Here's the drawing with two shaded views (mm, measured from the low corner). I have some questions. A direction names the side the tool comes from. Coordinates: 2 decimals unless noted, no trailing zeros. Loops run counter-clockwise (first coordinate to the right, second up) from the corner with the lowest first, then second, coordinate; pieces in that order, holes last. Notation, with made-up numbers: (80, 50.5) - (123, 50.5) arc R21 ccw to (123, 88.5) - close; hole circle Ø2 at (-35.75, 80). An arc over 180 degrees is marked (long way). Use a Markdown table: item, result.
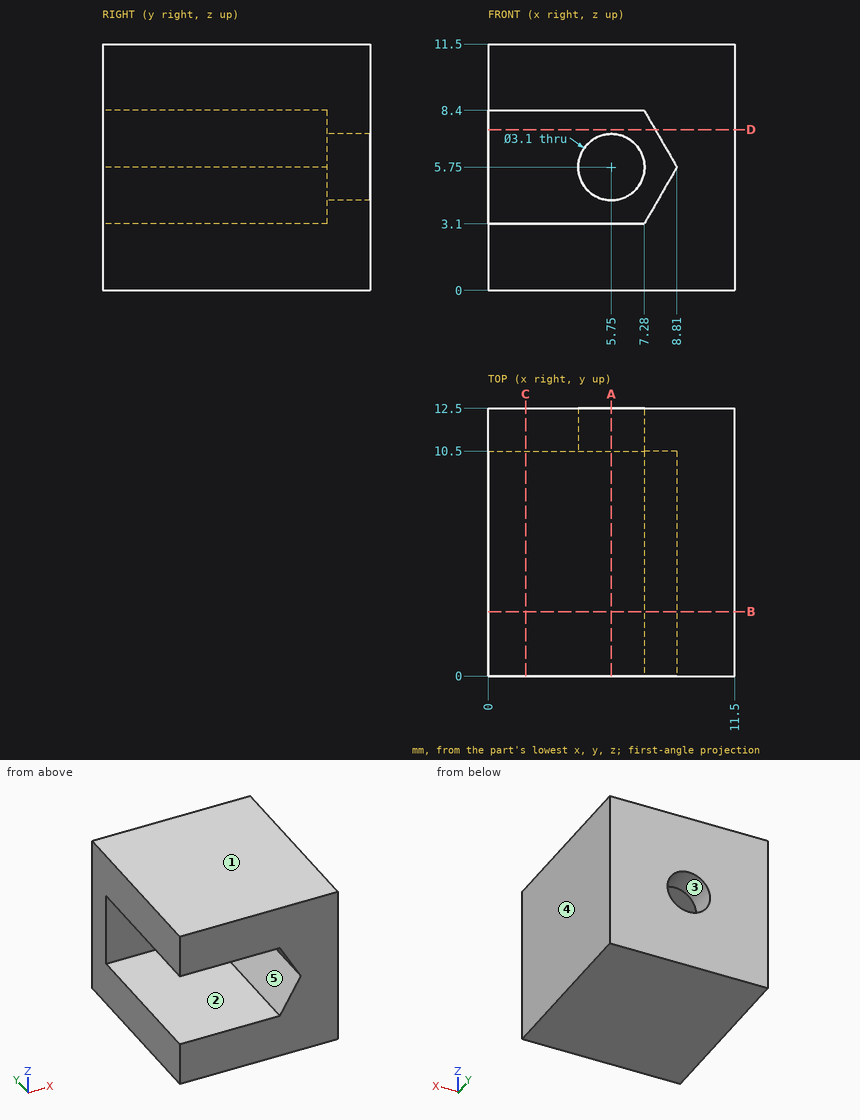
Q1. If we mould it in two halves opening along X, with no side actions, what happens to the marked faces 3, 4 and 5? For each: pulls with the +X half, pulls with the -X half, needs draft (parallel to the pull), parting line crosses it, or undercut.
Check values:
| item | result |
|---|---|
| face 3 | undercut |
| face 4 | pulls with the +X half |
| face 5 | pulls with the -X half |
Q2. Will these pins go through, and if not, where does the flat tip stop? P1, Ø3, axis at x = 5.5, y = 10, coming from the -Z side; P2, Ø1, axis at y = 9, z = 4.5, coming from the -X side.
Check values:
| item | result |
|---|---|
| P1 | z = 0 |
| P2 | x = 7.8 |
Q3. Which directions (+Z, -Z, +X, -X, +Y, -Y) give clear straight access to the entire face, cutting with the end or side of a thin tool? Please do the marked faces 1 and 2.
Check values:
| item | result |
|---|---|
| face 1 | +Z, +X, -X, +Y, -Y |
| face 2 | -X, -Y |
Q4. I want a section at A-A, the plane x = 5.75. Write out the boundary of the cut face in (y, z), then the cut area to 3 significant figures.
Check values:
| item | result |
|---|---|
| outline | (0, 0) - (12.5, 0) - (12.5, 4.2) - (10.5, 4.2) - (10.5, 3.1) - (0, 3.1) - close; (0, 8.4) - (10.5, 8.4) - (10.5, 7.3) - (12.5, 7.3) - (12.5, 11.5) - (0, 11.5) - close |
| area | 81.9 mm^2 |
Q5. I want a section at C-C, the plane x = 1.75. Write out the boundary of the cut face in (y, z).
Check values:
| item | result |
|---|---|
| outline | (0, 0) - (12.5, 0) - (12.5, 11.5) - (0, 11.5) - (0, 8.4) - (10.5, 8.4) - (10.5, 3.1) - (0, 3.1) - close |
Q6. Please list where these lines run through material, in increasing order: L1, parallel to X at y = 11.15, z = 5.75; L2, parallel to Z at x = 3.75, y = 5. Write a range as from..to.
Check values:
| item | result |
|---|---|
| L1 | 0..4.2, 7.3..11.5 |
| L2 | 0..3.1, 8.4..11.5 |
Q7. I want a section at D-D, the plane z = 7.5. Write out the boundary of the cut face in (x, y).
Check values:
| item | result |
|---|---|
| outline | (0, 10.5) - (7.8, 10.5) - (7.8, 0) - (11.5, 0) - (11.5, 12.5) - (0, 12.5) - close |
Q8. I want a section at B-B, the plane y = 3. Write out the boundary of the cut face in (x, z).
Check values:
| item | result |
|---|---|
| outline | (0, 0) - (11.5, 0) - (11.5, 11.5) - (0, 11.5) - (0, 8.4) - (7.28, 8.4) - (8.81, 5.75) - (7.28, 3.1) - (0, 3.1) - close |
